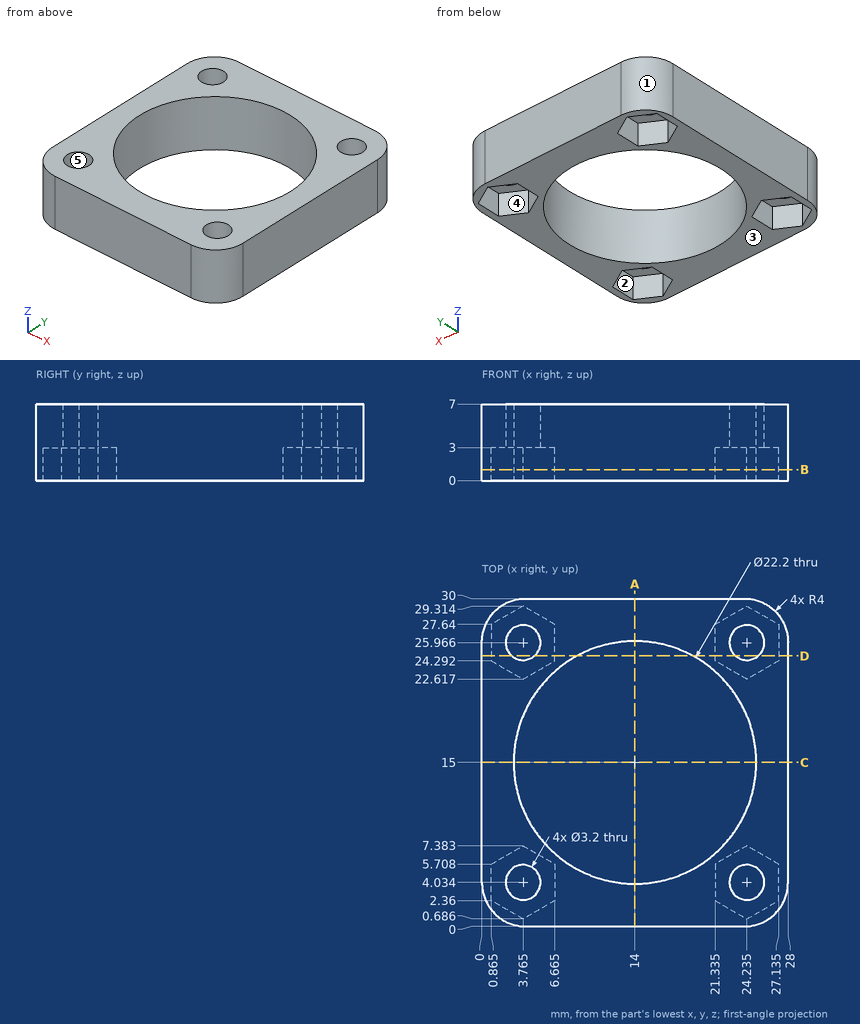
Can you work these out from the drawing? Everything is in mm from the part's minimum corner. A direction names the side the tool comes from. Give positions to 0.01 mm unless a question says otherwise; leave off trailing zeros. Order: outer loops, then holes, each group sorted by start corner. A loop starts at its lowest first (then second) coordinate and runs counter-clockwise, first axis right, second up.
Item 1: If we section it at C-C, the plane y = 15: Write out the boundary of the cut face in (x, z), plus the area to 3 significant figures.
Item 2: For the marked faces 4 and 5, which set-ups out of +Z, -Z, +X, -X, +Y, -Y let a thin tool reach every point of the face, with its end or its side?
Item 3: If we section it at D-D, the plane y = 24.75: Write out the boundary of the cut face in (x, z) (1 decimal).
Item 4: I need wall thicknesses on line 1 (X direction, y = 26.5, z = 1.5) (1 decimal); line 2 (X direction, y = 24.5, z = 1.25) (1 decimal); line 3 (X direction, y = 23.75, z = 1.75) (1 decimal). Which ranges of each line are inside material? Lowest first, please.
Item 5: I'm going to push flat-ended pins straight in: pin 1 (6.5 mm diameter, centred on x = 23.5, y = 3.5, fed in from -Z); pin 2 (5 mm diameter, centred on x = 24.23, y = 4.03, fed in from -Z); pin 3 (2.5 mm diameter, centred on x = 3.77, y = 25.97, fed in from +Z). Where does each tip first touch, or does it pass through?
Item 6: If we mould it in two halves opening along X, with no side actions, what happens to the marked faces 1, 2 and 3? For each: pulls with the +X half, pulls with the -X half, needs draft (parallel to the pull), parting line crosses it, or undercut.
Item 7: If we section it at B-B, the plane z = 1: Count the separate pieces of the cut face and the enclosed holes in it.
Item 8: If we section it at A-A, the plane x = 14: Write out the boundary of the cut face in (y, z), plus the area to 3 significant figures.
Values:
1. outline: (0, 0) - (2.9, 0) - (2.9, 7) - (0, 7) - close; (25.1, 0) - (28, 0) - (28, 7) - (25.1, 7) - close
1. area: 40.6 mm2
2. face 4: -Z
2. face 5: +Z, -Z
3. outline: (0, 0) - (0.9, 0) - (0.9, 3) - (2.7, 3) - (2.7, 7) - (0, 7) - close; (4.8, 3) - (6.7, 3) - (6.7, 0) - (8.7, 0) - (8.7, 7) - (4.8, 7) - close; (19.3, 0) - (21.3, 0) - (21.3, 3) - (23.2, 3) - (23.2, 7) - (19.3, 7) - close; (25.3, 3) - (27.1, 3) - (27.1, 0) - (28, 0) - (28, 7) - (25.3, 7) - close
4. line 1: x = 0 to 0.9, 6.7 to 21.3, 27.1 to 28
4. line 2: x = 0 to 0.9, 6.7 to 8.3, 19.7 to 21.3, 27.1 to 28
4. line 3: x = 0 to 1.8, 5.7 to 7.2, 20.8 to 22.3, 26.2 to 28
5. pin 1: stops at z = 0
5. pin 2: stops at z = 3
5. pin 3: passes through
6. face 1: pulls with the -X half
6. face 2: undercut
6. face 3: needs draft
7. separate pieces: 1
7. enclosed holes: 5
8. outline: (0, 0) - (3.9, 0) - (3.9, 7) - (0, 7) - close; (26.1, 0) - (30, 0) - (30, 7) - (26.1, 7) - close
8. area: 54.6 mm2
